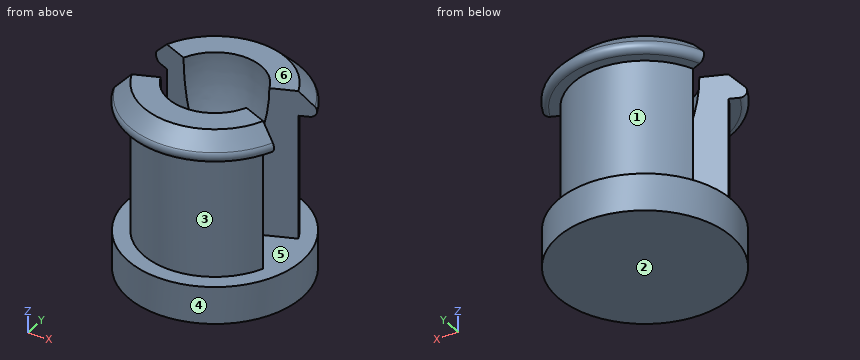
from build123d import *

# Parameters (mm, degrees)
SKETCH008_R         = 7
PAD002_DEPTH        = 3
REVOLUTION001_ANGLE = -135


with BuildPart() as part:
    # Sketch008 → Pad002 (new body)
    with BuildSketch(Plane.XY):
        Circle(SKETCH008_R)
    extrude(amount=-PAD002_DEPTH)

    # Sketch007 → Revolution001 (revolve)
    with BuildSketch(Plane(origin=(0, 0, 0), x_dir=(0.92388, -0.382683, 0), z_dir=(-0.382683, -0.92388, 0))):
        with BuildLine():
            Line((5.75, 0), (5.75, 10))
            Line((5.75, 10), (6.542893, 10))
            ThreePointArc((6.542893, 10), (7.004833, 10.308658), (6.896447, 10.853553))
            Line((6.896447, 10.853553), (5.75, 12))
            Line((5.75, 12), (3.75, 12))
            ThreePointArc((0, 3), (2.775, 7.125), (3.75, 12))
            Line((0, 0), (0, 3))
            Line((5.75, 0), (0, 0))
        make_face()
    revolution001 = revolve(axis=Axis((0, 0, 0), (0, 0, 1)), revolution_arc=REVOLUTION001_ANGLE)

    # Mirrored001: Revolution001 across XZ
    add(revolution001.mirror(Plane.XZ))


solid = part.part
Can you work these out from the model? Positions are in its coordinate system, mm. Face numbers are marked on the shaded views. A direction names the side the tool comes from. Give positions to 0.01 mm unless a question says otherwise; leave off trailing zeros. Answer as a JSON object with one key per item and string values. Group by question number.
Item 1: For the marked faces 1, 2 and 3, which set-ups out of +Z, -Z, +X, -X, +Y, -Y let a thin tool reach every point of the face, with its end or its side?
Item 2: I'm going to push flat-ended pins straight in: P1, Ø6, axis at x = 5.5, z = 1, coming from the -Y side; P2, Ø1.5, axis at x = -3.5, z = 1.5, coming from the +Y side; P3, Ø1.5, axis at y = -2, z = 6.5, coming from the -X side. Where does each tip first touch, or does it pass through?
Item 3: Please list where these lines run through material, in increasing order: line 1 (Y direction, x = -0.5, z = 3); line 2 (Y direction, x = 3, z = 10.25); line 3 (Z direction, x = 1, y = -0.25). Write a range as [from, to].
Item 4: We'd pull the mould along Z, two halves only. Please class the marked faces 4, 5 and 6: +Z half, -Z half, draft (parallel to the pull), parting line (faces both ways), or undercut.
Findings:
{
 "1": {"face 1": "+Y", "face 2": "-Z, +X, -X, +Y, -Y", "face 3": "-Y"},
 "2": {"P1": "stops at y = -6.47", "P2": "stops at y = 5.05", "P3": "stops at x = -5.31"},
 "3": {"line 1": "y = [-5.73, -0.21], [0.21, 5.73]", "line 2": "y = [-6.3, -2.04], [2.04, 6.3]", "line 3": "z = [-3, 0]"},
 "4": {"face 4": "draft", "face 5": "undercut", "face 6": "+Z half"}
}
